Part print with two shaded views. Sizes in mm from the minimum x, y, z corner. Give positions to 0.01 mm unless a question says otherwise; leave off trailing zeros. Loops run counter-clockwise (first coordinate to the right, second up) from the corner with the lowest first, then second, coordinate; pieces in that order, holes last. Notation, with made-up numbers: M 43.5,-13.75 L 76.5,-13.75 A22 ccw 76.5,25.25 Z; hole C 12.25,21 d7. An arc over 180 degrees is marked long. Answer as a JSON object with one key per item and string values. Group by question number.
1. Slice it at A-A (x = 151.5). List the corners of the cut face in (y, z).
2. Drill centre lines: line 1 along Z through (x, y) = (111, 2.1); line 2 along X through (y, z) = (2.5, 14.5). Where is each one in solid material? Low to high. Write a range as [from, to].
3. Drop flat-ended pins along their axis: pin 1 Ø1.5 at (y, z) = (2, 39) entering from -X; pin 2 Ø0.9 at (y, z) = (1.5, 4) entering from +X. Give the stop position or say it passes through.
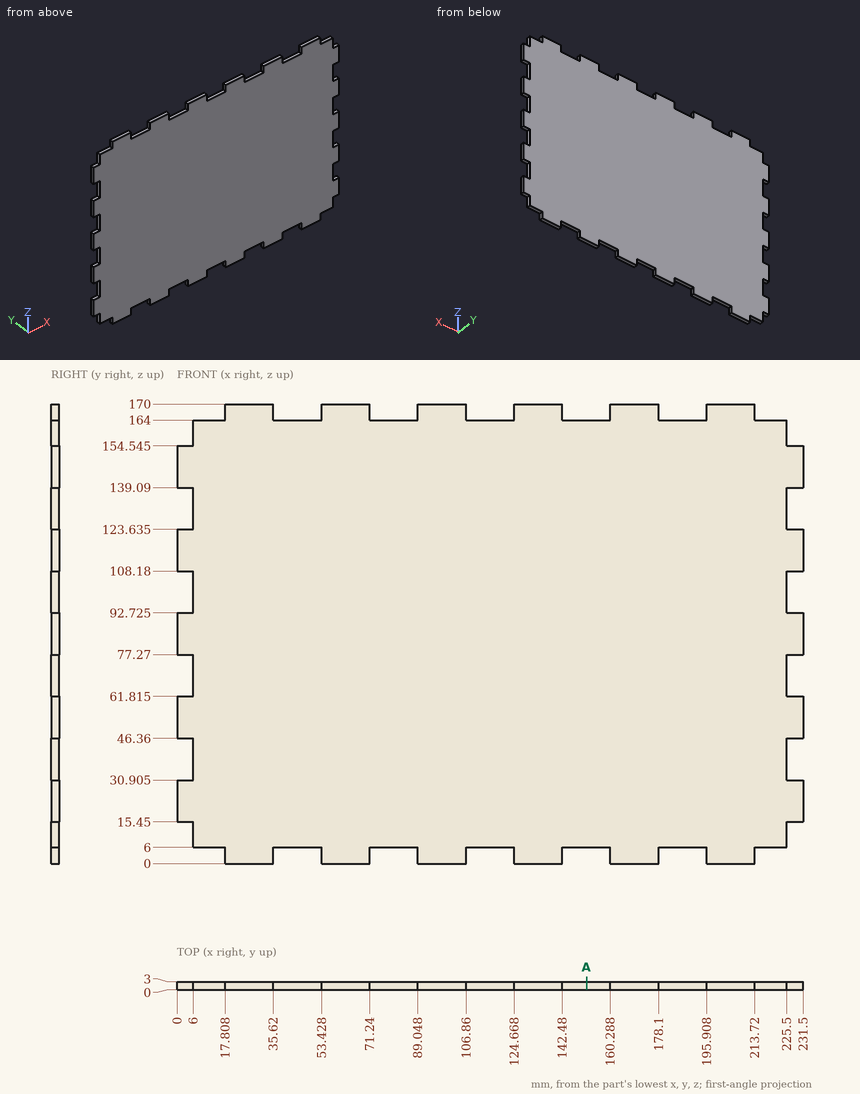
Established:
{
 "1": {"outline": "M 0,6 L 3,6 L 3,164 L 0,164 Z"},
 "2": {"line 1": "z = [6, 164]", "line 2": "x = [6, 225.5]"},
 "3": {"pin 1": "stops at x = 6", "pin 2": "stops at x = 213.72"}
}
